from build123d import *

# Parameters (mm, degrees)
BOSS_EXTRUDE1_DEPTH                  = 158.8516
F_10_32_TAPPED_HOLE1_D               = 4.0386
F_10_32_TAPPED_HOLE1_DEPTH           = 12.02944
F_10_32_TAPPED_HOLE1_TIP             = 1.213317848
F_10_32_TAPPED_HOLE1_ON_FACE_2_D     = 4.0386
F_10_32_TAPPED_HOLE1_ON_FACE_2_DEPTH = 12.02944
F_10_32_TAPPED_HOLE1_ON_FACE_2_TIP   = 1.213317848


with BuildPart() as part:
    # Sketch1 → Boss-Extrude1 (new, symmetric)
    with BuildSketch(Plane.XY):
        with BuildLine():
            ThreePointArc((6.35, 2.590301913), (5.939202219, 3.429), (5.41826726, 4.204110358))
            Line((5.41826726, 4.204110358), (0.93173274, 6.79441227))
            ThreePointArc((0.93173274, 6.79441227), (0, 6.858), (-0.93173274, 6.79441227))
            Line((-0.93173274, 6.79441227), (-5.41826726, 4.204110358))
            ThreePointArc((-5.41826726, 4.204110358), (-5.939202219, 3.429), (-6.35, 2.590301913))
            Line((-6.35, 2.590301913), (-6.35, -2.590301913))
            ThreePointArc((-6.35, -2.590301913), (-5.939202219, -3.429), (-5.41826726, -4.204110358))
            Line((-5.41826726, -4.204110358), (-0.93173274, -6.79441227))
            ThreePointArc((-0.93173274, -6.79441227), (0, -6.858), (0.93173274, -6.79441227))
            Line((0.93173274, -6.79441227), (5.41826726, -4.204110358))
            ThreePointArc((5.41826726, -4.204110358), (5.939202219, -3.429), (6.35, -2.590301913))
            Line((6.35, -2.590301913), (6.35, 2.590301913))
        make_face()
    extrude(amount=BOSS_EXTRUDE1_DEPTH, both=True)

    # #10-32 Tapped Hole1
    with Locations(Plane(origin=(0, 0, -158.8516), x_dir=(-1, 0, 0), z_dir=(0, 0, -1))):
        with Locations((0, 0)):
            Hole(F_10_32_TAPPED_HOLE1_D / 2, depth=F_10_32_TAPPED_HOLE1_DEPTH)
            with Locations((0, 0, -(F_10_32_TAPPED_HOLE1_DEPTH + F_10_32_TAPPED_HOLE1_TIP / 2))):  # 118° drill point
                Cone(0, F_10_32_TAPPED_HOLE1_D / 2, F_10_32_TAPPED_HOLE1_TIP, mode=Mode.SUBTRACT)

    # #10-32 Tapped Hole1 on face 2
    with Locations(Plane.XY.offset(158.8516)):
        with Locations((0, 0)):
            Hole(F_10_32_TAPPED_HOLE1_ON_FACE_2_D / 2, depth=F_10_32_TAPPED_HOLE1_ON_FACE_2_DEPTH)
            with Locations((0, 0, -(F_10_32_TAPPED_HOLE1_ON_FACE_2_DEPTH + F_10_32_TAPPED_HOLE1_ON_FACE_2_TIP / 2))):  # 118° drill point
                Cone(0, F_10_32_TAPPED_HOLE1_ON_FACE_2_D / 2, F_10_32_TAPPED_HOLE1_ON_FACE_2_TIP, mode=Mode.SUBTRACT)


solid = part.part
Work out the finished part from the listing and answer in its coordinate system (mm). Coordinates: 2 decimals unless noted, no trailing zeros. Write each loop counter-clockwise with the first axis right and the second up, starting at its lowest first coordinate (ties: lowest second). Pieces come first, ordered by that corner, then holes.
1. The part is cut by section A-A, the plane z = -55. Write down the section's boundary in (x, y).
Results list:
outline: (-6.35, -2.59) arc R6.86 ccw to (-5.42, -4.2) - (-0.93, -6.79) arc R6.86 ccw to (0.93, -6.79) - (5.42, -4.2) arc R6.86 ccw to (6.35, -2.59) - (6.35, 2.59) arc R6.86 ccw to (5.42, 4.2) - (0.93, 6.79) arc R6.86 ccw to (-0.93, 6.79) - (-5.42, 4.2) arc R6.86 ccw to (-6.35, 2.59) - close
2. Consider line 1 along X through (y, z) = (0, 152); line 2 along Y through (x, z) = (0, 154.5); line 3 along Y through (x, z) = (-1, -0.5) (3 decimals). Determine where each line is inside the solid, lowest interval first.
Results list:
line 1: x = -6.35 to -2.02, 2.02 to 6.35
line 2: y = -6.86 to -2.02, 2.02 to 6.86
line 3: y = -6.755 to 6.755
3. Flat-ended cylindrical pins translate along their axes: pin 1 (3 mm diameter, centred on y = -5, z = 99.5, fed in from +X); pin 2 (3 mm diameter, centred on x = 0, y = 0, fed in from -Z); pin 3 (2 mm diameter, centred on y = -4, z = -9.5, fed in from +X). Find the tip coordinate at first contact, or state that the pin passes through.
Results list:
pin 1: stops at x = 5.9
pin 2: stops at z = -146.51
pin 3: stops at x = 6.17
